from build123d import *

# Parameters (mm, degrees)
SKETCH2_R          = 1.5
CUT_EXTRUDE1_DEPTH = 9.185352772


with BuildPart() as part:
    # Sketch1 → Revolve1 (revolve)
    with BuildSketch(Plane(origin=(0, 0, 0), x_dir=(1, 0, 0), z_dir=(0, 1, 0))):
        with BuildLine():
            Line((0, 0), (0, 7))
            Line((0, 7), (2.5, 7))
            Line((2.5, 7), (1.6, 6.25))
            Line((1.6, 6.25), (1.6, 6.037715508))
            ThreePointArc((1.6, 6.037715508), (3, 3.5), (1.6, 0.962284492))
            Line((1.6, 0.962284492), (1.6, 0.75))
            Line((1.6, 0.75), (2.5, 0))
            Line((2.5, 0), (0, 0))
        make_face()
    revolve(axis=Axis((0, 0, 0), (0, 0, -1)))

    # Sketch2 → Cut-Extrude1 (cut, through all)
    with BuildSketch(Plane.XY):
        Circle(SKETCH2_R)
    extrude(amount=-CUT_EXTRUDE1_DEPTH, mode=Mode.SUBTRACT)


solid = part.part
CAD build for the part. Positions are in the model's coordinates, mm. Round coordinates to 2 decimals unless told otherwise and drop trailing zeros. Loops run counter-clockwise (first coordinate to the right, second up) from the corner with the lowest first, then second, coordinate; pieces in that order, holes last. Notation, with made-up numbers: (-39, 1) - (-14, 1) arc R15 cw to (-14, 27) - close; hole circle Ø7 at (57.25, -8). An arc over 180 degrees is marked (long way). Put each result on its own line as item: value.
1. Slice it at A-A on y = 0. List the corners of the cut face in (x, z), and give its area (3 significant figures).
Geometry check:
outline: (-2.5, -7) - (-1.5, -7) - (-1.5, 0) - (-2.5, 0) - (-1.6, -0.75) - (-1.6, -0.96) arc R3 ccw to (-1.6, -6.04) - (-1.6, -6.25) - close; (1.5, -7) - (2.5, -7) - (1.6, -6.25) - (1.6, -6.04) arc R3 ccw to (1.6, -0.96) - (1.6, -0.75) - (2.5, 0) - (1.5, 0) - close
area: 12.8 mm²
2. Slice it at C-C on z = -4.5. List the corners of the cut face in (x, y).
Geometry check:
outline: circle Ø5.66 at (0, 0); hole circle Ø3 at (0, 0)
3. Pin check, flat tip, straight feed: P1, Ø1, axis at y = 1, z = -5.5, coming from the -X side. Stop position of the tip, or through.
Geometry check:
P1: x = -2.45
4. Wall check: line 1 (Z direction, x = -1.4, y = 1.8); line 2 (Z direction, x = 0.8, y = -1.9); line 3 (Y direction, x = -1.15, z = -6). Give the ranges that are in metal, low to high.
Geometry check:
line 1: -7 to -6.82, -5.45 to -1.55, -0.18 to 0
line 2: -7 to -6.63, -5.68 to -1.32, -0.37 to 0
line 3: -1.19 to -0.96, 0.96 to 1.19
5. Two-plate mould, pull along Y, no slides. Class faces 1 (the cylindrical face through (-1.5, 0.07, -3.45)), 2 (the flat face through (-2, 0, -7)): released by +Y, released by -Y, zero draft, split by the parting line, or undercut.
Geometry check:
face 1: undercut
face 2: zero draft
6. Slice it at D-D on x = 1.9. Give the number of separate pieces and of enclosed holes in the cut face, and give its area (3 significant figures).
Geometry check:
separate pieces: 3
enclosed holes: 0
area: 19.0 mm²
